from build123d import *

# Parameters (mm, degrees)
EXTRUDE_1_DEPTH          = 5
EXTRUDE_1_DEPTH_BACK     = 5
SKETCH_1_R               = 12
CUT_EXTRUDE_1_DEPTH      = 10
CUT_EXTRUDE_1_DEPTH_BACK = 10
SKETCH_2_R               = 3


with BuildPart() as part:
    # 草图1 → 凸台-拉伸1 (new, two sides: drawn at the far end of the back side and taken through both)
    with BuildSketch(Plane.XY.offset(-EXTRUDE_1_DEPTH_BACK)):
        with BuildLine():
            Line((21.997045256, -12.7), (24.768326548, -14.3))
            ThreePointArc((24.768326548, -14.3), (26.42295463, -10.944746166), (27.625478632, -7.40222469))
            Line((27.625478632, -7.40222469), (24.534515988, -6.574003746))
            ThreePointArc((24.534515988, -6.574003746), (25.182699479, -3.315365282), (25.4, 0))
            Line((25.4, 0), (28.6, 0))
            ThreePointArc((28.6, 0), (28.355323035, 3.733049097), (27.625478632, 7.40222469))
            Line((27.625478632, 7.40222469), (24.534515988, 6.574003746))
            ThreePointArc((24.534515988, 6.574003746), (23.466540126, 9.720159182), (21.997045256, 12.7))
            Line((21.997045256, 12.7), (24.768326548, 14.3))
            ThreePointArc((24.768326548, 14.3), (22.689905532, 17.41057687), (20.223253942, 20.223253942))
            Line((20.223253942, 20.223253942), (17.960512242, 17.960512242))
            ThreePointArc((17.960512242, 17.960512242), (15.462540297, 20.151174843), (12.7, 21.997045256))
            Line((12.7, 21.997045256), (14.3, 24.768326548))
            ThreePointArc((14.3, 24.768326548), (10.944746166, 26.42295463), (7.40222469, 27.625478632))
            Line((7.40222469, 27.625478632), (6.574003746, 24.534515988))
            ThreePointArc((6.574003746, 24.534515988), (3.315365282, 25.182699479), (0, 25.4))
            Line((0, 25.4), (0, 28.6))
            ThreePointArc((0, 28.6), (-3.733049097, 28.355323035), (-7.40222469, 27.625478632))
            Line((-7.40222469, 27.625478632), (-6.574003746, 24.534515988))
            ThreePointArc((-6.574003746, 24.534515988), (-9.720159182, 23.466540126), (-12.7, 21.997045256))
            Line((-12.7, 21.997045256), (-14.3, 24.768326548))
            ThreePointArc((-14.3, 24.768326548), (-17.41057687, 22.689905532), (-20.223253942, 20.223253942))
            Line((-20.223253942, 20.223253942), (-17.960512242, 17.960512242))
            ThreePointArc((-17.960512242, 17.960512242), (-20.151174843, 15.462540297), (-21.997045256, 12.7))
            Line((-21.997045256, 12.7), (-24.768326548, 14.3))
            ThreePointArc((-24.768326548, 14.3), (-26.42295463, 10.944746166), (-27.625478632, 7.40222469))
            Line((-27.625478632, 7.40222469), (-24.534515988, 6.574003746))
            ThreePointArc((-24.534515988, 6.574003746), (-25.182699479, 3.315365282), (-25.4, 0))
            Line((-25.4, 0), (-28.6, 0))
            ThreePointArc((-28.6, 0), (-28.355323035, -3.733049097), (-27.625478632, -7.40222469))
            Line((-27.625478632, -7.40222469), (-24.534515988, -6.574003746))
            ThreePointArc((-24.534515988, -6.574003746), (-23.466540126, -9.720159182), (-21.997045256, -12.7))
            Line((-21.997045256, -12.7), (-24.768326548, -14.3))
            ThreePointArc((-24.768326548, -14.3), (-22.689905532, -17.41057687), (-20.223253942, -20.223253942))
            Line((-20.223253942, -20.223253942), (-17.960512242, -17.960512242))
            ThreePointArc((-17.960512242, -17.960512242), (-15.462540297, -20.151174843), (-12.7, -21.997045256))
            Line((-12.7, -21.997045256), (-14.3, -24.768326548))
            ThreePointArc((-14.3, -24.768326548), (-10.944746166, -26.42295463), (-7.40222469, -27.625478632))
            Line((-7.40222469, -27.625478632), (-6.574003746, -24.534515988))
            ThreePointArc((-6.574003746, -24.534515988), (-3.315365282, -25.182699479), (0, -25.4))
            Line((0, -25.4), (0, -28.6))
            ThreePointArc((0, -28.6), (3.733049097, -28.355323035), (7.40222469, -27.625478632))
            Line((7.40222469, -27.625478632), (6.574003746, -24.534515988))
            ThreePointArc((6.574003746, -24.534515988), (9.720159182, -23.466540126), (12.7, -21.997045256))
            Line((12.7, -21.997045256), (14.3, -24.768326548))
            ThreePointArc((14.3, -24.768326548), (17.41057687, -22.689905532), (20.223253942, -20.223253942))
            Line((20.223253942, -20.223253942), (17.960512242, -17.960512242))
            ThreePointArc((17.960512242, -17.960512242), (20.151174843, -15.462540297), (21.997045256, -12.7))
        make_face()
        Circle(SKETCH_1_R, mode=Mode.SUBTRACT)
    extrude(amount=EXTRUDE_1_DEPTH + EXTRUDE_1_DEPTH_BACK)

    # 草图2 → 切除-拉伸1 (cut, two sides: drawn at the far end of the back side and taken through both)
    with BuildSketch(Plane.XY.offset(-CUT_EXTRUDE_1_DEPTH_BACK)):
        with Locations((18, 0)):
            Circle(SKETCH_2_R)
        with Locations((0, -18)):
            Circle(SKETCH_2_R)
        with Locations((-18, 0)):
            Circle(SKETCH_2_R)
        with Locations((0, 18)):
            Circle(SKETCH_2_R)
    extrude(amount=CUT_EXTRUDE_1_DEPTH + CUT_EXTRUDE_1_DEPTH_BACK, mode=Mode.SUBTRACT)


solid = part.part
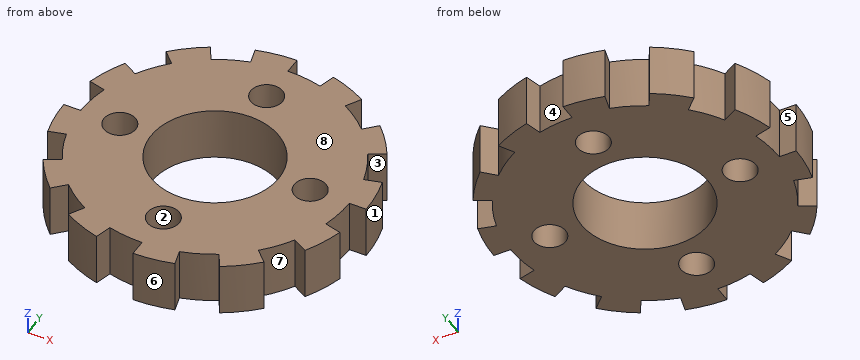
Work out the finished part from the listing and answer in its coordinate system (mm). Face numbers are marked on the shaded views. A direction names the side the tool comes from. Coordinates: 2 decimals unless noted, no trailing zeros. Order: outer loops, then holes, each group sorted by start corner. A loop starts at its lowest first (then second) coordinate and runs counter-clockwise, first axis right, second up. Notation, with made-up numbers: (37.5, 87) - (87.5, 87) arc R9 ccw to (87.5, 103) - close; hole circle Ø10 at (9, -22.75). An arc over 180 degrees is marked (long way). Put each result on its own line as item: value. Start each with the question number.
1) Find section A-A (x = -16.5). Give the vertices of the cut face in (y, z).
2) Flat-ended cylindrical pins translate along their axes: pin 1 (3.5 mm diameter, centred on x = 18, y = 0, fed in from +Z) (3 decimals); pin 2 (1 mm diameter, centred on x = 26.5, z = 1.5, fed in from -Y); pin 3 (1 mm diameter, centred on y = -22, z = 0.5, fed in from +X); pin 4 (6 mm diameter, centred on x = 3.5, z = 1, fed in from +Y). Find the tip coordinate at first contact, or state that the pin passes through.
3) Find the intervals of material crossed by line 1 (X direction, y = -19, z = -2.5); line 2 (Y direction, x = 20, z = -2.75); line 3 (X direction, y = -13, z = 4.75), in increasing order. Write a range as from..to.
4) For the marked faces 1, 2, 3, 4 and 5, determine the directions among +Z, -Z, +X, -X, +Y, -Y from which every point of the face is accessible in a straight line to the end or side of a thin tool.
5) Find section C-C (z = 1.25). State how many separate pieces and enclosed holes the cut face has, plus the area to 3 significant figures.
6) Find section B-B (y = 4). Give the vertices of the cut face in (x, z), plus the area to 3 significant figures.
7) For a pull along Y with two mould halves and no side action, classify the marked faces 6, 7 and 8 as released by +Y, released by -Y, zero draft, split by the parting line, or undercut.
Results list:
1. outline: (-19.31, -5) - (-2.6, -5) - (-2.6, 5) - (-19.31, 5) - close; (2.6, -5) - (23.36, -5) - (23.36, 5) - (2.6, 5) - close
2. pin 1: passes through
2. pin 2: stops at y = -11.91
2. pin 3: stops at x = 18.86
2. pin 4: stops at y = 25.4
3. line 1: x = -21.38..-19, -16.86..-2.83, 2.83..19
3. line 2: y = -20.44..-20, -15.66..-2.24, 2.24..20
3. line 3: x = -22.52..21.82, 22.52..25.47
4. face 1: +Z, -Z, +X, +Y
4. face 2: +Z, -Z
4. face 3: +Z, -Z, +X
4. face 4: +Z, -Z, +Y
4. face 5: +Z, -Z, -X
5. separate pieces: 1
5. enclosed holes: 5
5. area: 1,730 mm^2
6. outline: (-25.08, -5) - (-11.31, -5) - (-11.31, 5) - (-25.08, 5) - close; (11.31, -5) - (28.32, -5) - (28.32, 5) - (11.31, 5) - close
6. area: 308 mm^2
7. face 6: released by -Y
7. face 7: undercut
7. face 8: zero draft
